from build123d import *

# Parameters (mm, degrees)
F0_R      = 12.5
F1_DEPTH  = 80
F2_R      = 5
F3_ANGLE  = 60
F4_R      = 6.5
F5_DEPTH  = 45
F6_R      = 5.4
F7_DEPTH  = 10
F8_R      = 5
F9_ANGLE  = 30
F10_DEPTH = 5
F11_R     = 22.5
F11_R_2   = 5
F12_DEPTH = 100
F13_SIZE  = 10
F14_SIZE  = 10


with BuildPart() as f1:
    # F0 (on Right) → F1 (new body)
    with BuildSketch(Plane.YZ):
        Circle(F0_R)
    extrude(amount=F1_DEPTH)

    # F2 (on face) → F3 (revolve)
    with BuildSketch(Plane.YZ.offset(80)):
        Circle(F2_R)
    revolve(axis=Axis((80, 12.480231002, -12.5), (0, 1, 0)), revolution_arc=F3_ANGLE)

    # F4 (on face) → F5 (join)
    with BuildSketch(Plane(origin=(25.4126587737, 0, -44.0160161514), x_dir=(0.8660254038, 0, 0.5), z_dir=(0.5, 0, -0.8660254038))):
        with Locations((75.5320323028, 0)):
            Circle(F4_R)
    extrude(amount=F5_DEPTH)

    # F6 (on face) → F7 (join)
    with BuildSketch(Plane(origin=(0, 0, 0), x_dir=(0, -1, 0), z_dir=(-1, 0, 0))):
        Circle(F6_R)
    extrude(amount=F7_DEPTH)

    # F8 (on face) → F9 (revolve)
    with BuildSketch(Plane(origin=(47.9126587737, 0, -82.9871593217), x_dir=(0.8660254038, 0, 0.5), z_dir=(0.5, 0, -0.8660254038))):
        with Locations((75.5320323028, 0)):
            Circle(F8_R)
    revolve(axis=Axis((106.1030469169, 6.7506376654, -49.3909230629), (0, 1, 0)), revolution_arc=F9_ANGLE)

    # F10 (add): a face of the model
    f10_faces = [f1.faces().sort_by_distance(p)[0] for p in [
        (114.4426067022, 0, -49.3909230629),
    ]]
    extrude(f10_faces, amount=F10_DEPTH)

    # F11 (on face) → F12 (join)
    with BuildSketch(Plane(origin=(0, 0, -54.3909230629), x_dir=(1, 0, 0), z_dir=(0, 0, -1))):
        with Locations((114.4426067022, 0)):
            Circle(F11_R)
        with Locations((114.4426067022, 0)):
            Circle(F11_R_2, mode=Mode.SUBTRACT)
        with Locations((114.4426067022, 0)):
            Circle(F11_R_2)
    extrude(amount=F12_DEPTH)

    # F13
    f13_edges = [f1.edges().sort_by_distance(p)[0] for p in [
        (91.942607, 0, -54.390923),
    ]]
    chamfer(f13_edges, length=F13_SIZE)

    # F14
    f14_edges = [f1.edges().sort_by_distance(p)[0] for p in [
        (91.942607, 0, -154.390923),
    ]]
    chamfer(f14_edges, length=F14_SIZE)


solid = f1.part
The listing builds one solid part. Answer for the finished solid, in the listing's coordinates (mm). A direction names the side the tool comes from. Give positions to 0.01 mm unless a question says otherwise; leave off trailing zeros. Write each loop counter-clockwise with the first axis right and the second up, starting at its lowest first coordinate (ties: lowest second). Pieces come first, ordered by that corner, then holes. Notation, with made-up numbers: (-9, -16) -> (29, -16) arc R24 cw to (29, 21) -> close; hole circle Ø10 at (70.5, 28). An arc over 180 degrees is marked (long way). Use a Markdown table: item, result.
(1) Section B-B, the plane z = -86.5 is taken. Determine the outline of the cut face in (x, y).
Return value:
| item | result |
|---|---|
| outline | circle Ø45 at (114.44, 0) |
(2) Flat-ended cylindrical pins translate along their axes: P1, Ø10, axis at y = 12.5, z = -88.5, coming from the -X side; P2, Ø8, axis at x = 106, z = -29, coming from the -Y side; P3, Ø20, axis at y = 6, z = -0.5, coming from the +X side. Find the tip coordinate at first contact, or state that the pin passes through.
Return value:
| item | result |
|---|---|
| P1 | x = 93.23 |
| P2 | y = -6.5 |
| P3 | x = 99.96 |
(3) Section C-C, the plane x = 59 is taken. Determine the outline of the cut face in (y, z).
Return value:
| item | result |
|---|---|
| outline | circle Ø25 at (0, 0) |
(4) For faces 1 (the flat face through (0, 3, -5)), 2 (the flat face through (114.3, 5.4, -54.391)), 3 (the flat face through (-10, 0, 0)), determine the directions among +Z, -Z, +X, -X, +Y, -Y from which every point of the face is accessible in a straight line to the end or side of a thin tool.
Return value:
| item | result |
|---|---|
| face 1 | -X |
| face 2 | none |
| face 3 | +Z, -Z, -X, +Y, -Y |
(5) Find the intervals of material crossed by probe 1 along X at (y, z) = (-8.5, 2); probe 2 along Y at (x, z) = (114, -46.5); probe 3 along Z at (x, y) = (99, 3.5), in increasing order. Write a range as from..to.
Return value:
| item | result |
|---|---|
| probe 1 | 0..80 |
| probe 2 | -5..5 |
| probe 3 | -151.06..-57.73, -31.36..-9.45 |
(6) Determine the mould class of faces 4 (the flat face through (114, 0, -154.391)), 5 (the flat face through (89.13, 4.78, -7.23)), 6 (the flat face through (80, -0.2, -5.4)) for opening direction Z: released by +Z, released by -Z, zero draft, split by the parting line, or undercut.
Return value:
| item | result |
|---|---|
| face 4 | released by -Z |
| face 5 | undercut |
| face 6 | zero draft |
